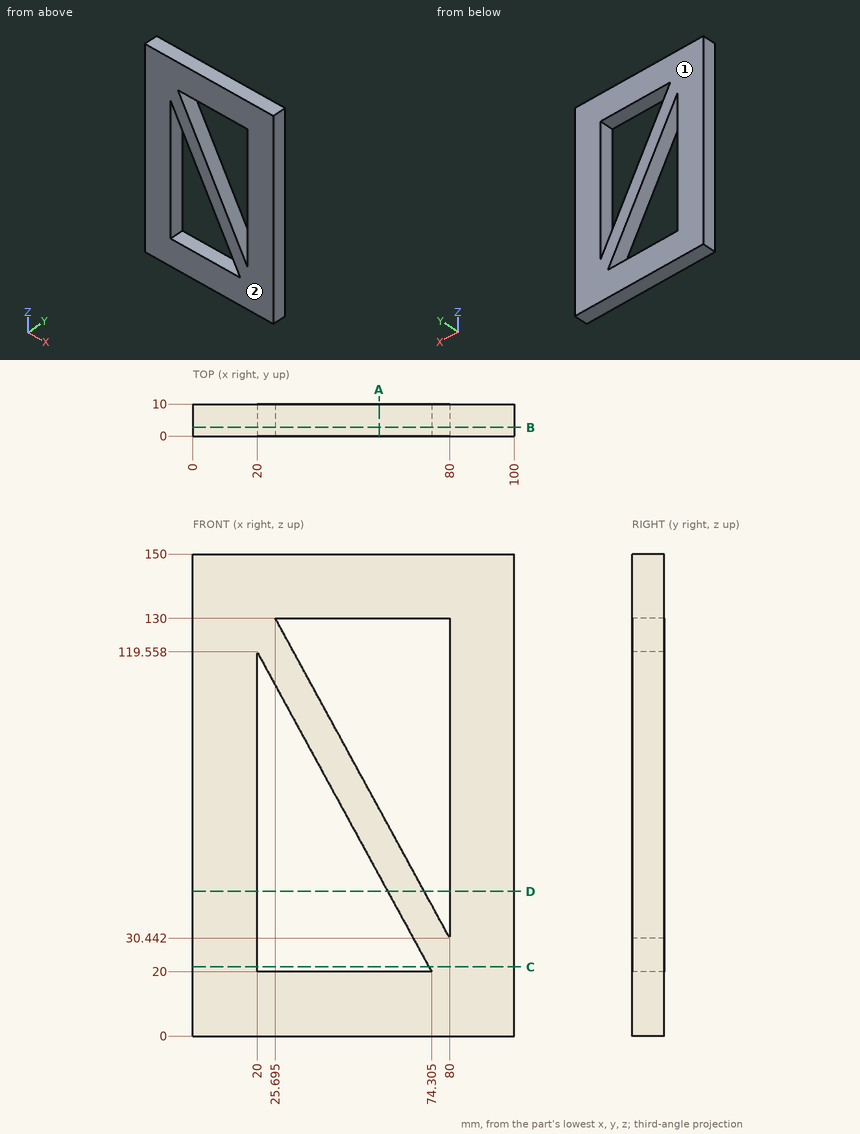
For this review, use the dimensioned drawing (mm, ordinates from the lowest corner) and the shaded views. Round coordinates to 2 decimals unless told otherwise and drop trailing zeros. Order: outer loops, then holes, each group sorted by start corner. A loop starts at its lowest first (then second) coordinate and runs counter-clockwise, first axis right, second up. Notation, with made-up numbers: (-11, 52) -> (29, 52) arc R25 cw to (29, 84) -> close; hole circle Ø5 at (-33, 27.5). An arc over 180 degrees is marked (long way). Write item = value, one per line. Start each with the question number.
Item 1: Consider section A-A on x = 58. Write out the cut boundary in (y, z) (1 decimal), plus the area to 3 significant figures.
Item 2: Consider section D-D on z = 45. Write out the cut boundary in (x, y), plus the area to 3 significant figures.
Item 3: Mouldability with a two-part tool opening along Y and no side actions: class the marked faces 1 and 2 as released by +Y, released by -Y, zero draft, split by the parting line, or undercut.
Item 4: Consider section B-B on y = 2.75. Write out the cut boundary in (x, z) (1 decimal), plus the area to 3 significant figures.
Item 5: Consider section C-C on z = 21.5. Write out the cut boundary in (x, y), plus the area to 3 significant figures.
Item 6: For line 1 along Z through (x, y) = (37.5, 8.5) (1 decimal); line 2 along Z through (x, y) = (58, 5) (1 decimal); line 3 along X through (y, z) = (9, 108) (1 decimal), list the stretches that pass through material, from the lowest coordinate up.
Conclusion:
q1.outline = (0, 0) -> (10, 0) -> (10, 20) -> (0, 20) -> close; (0, 49.9) -> (10, 49.9) -> (10, 70.8) -> (0, 70.8) -> close; (0, 130) -> (10, 130) -> (10, 150) -> (0, 150) -> close
q1.area = 609 mm2
q2.outline = (0, 0) -> (20, 0) -> (20, 10) -> (0, 10) -> close; (60.67, 0) -> (72.06, 0) -> (72.06, 10) -> (60.67, 10) -> close; (80, 0) -> (100, 0) -> (100, 10) -> (80, 10) -> close
q2.area = 514 mm2
q3.face_1 = released by +Y
q3.face_2 = released by -Y
q4.outline = (0, 0) -> (100, 0) -> (100, 150) -> (0, 150) -> close; hole (20, 20) -> (74.3, 20) -> (20, 119.6) -> close; hole (25.7, 130) -> (80, 30.4) -> (80, 130) -> close
q4.area = 9,590 mm2
q5.outline = (0, 0) -> (20, 0) -> (20, 10) -> (0, 10) -> close; (73.49, 0) -> (100, 0) -> (100, 10) -> (73.49, 10) -> close
q5.area = 465 mm2
q6.line_1 = 0 to 20, 87.5 to 108.4, 130 to 150
q6.line_2 = 0 to 20, 49.9 to 70.8, 130 to 150
q6.line_3 = 0 to 20, 26.3 to 37.7, 80 to 100
